Geometry: final body of the model. Coordinates: model frame, mm. A direction names the side the tool comes from. Coordinates: 2 decimals unless noted, no trailing zeros. Write each loop counter-clockwise with the first axis right and the second up, starting at its lowest first coordinate (ties: lowest second). Pieces come first, ordered by that corner, then holes. Notation, with made-up numbers: (-26.75, 8.25) - (13.25, 8.25) arc R18 cw to (13.25, 40.25) - close; hole circle Ø1 at (0, 51). An arc over 180 degrees is marked (long way). Answer as a JSON object with one key per item and string values. Group by question number.
Item 1: Line query: line 1 along Y through (x, z) = (8, 1.25); line 2 along X through (y, z) = (-14.5, 9.25); line 3 along Y through (x, z) = (1.5, 7.5). Output: solid intervals per line, ascending. Write a range as from..to.
Item 2: First-contact query: pin 1 Ø2 at (x, z) = (8.5, 7) entering from -Y; pin 2 Ø6.5 at (y, z) = (-8.5, 7) entering from +X. Flat tips, straight axial feed; report the tip coordinate or a pass-through.
Item 3: Mould query, pull axis Z, two halves, no side actions, for faces 3 (the flat face through (1, -5, 0)), 4 (the flat face through (0, -11.5, 4.8)), 5 (the cylindrical face through (0.867, -13.675, 4.249)). Classes: pulls with the +Z half, pulls with the -Z half, needs draft (parallel to the pull), parting line crosses it, or undercut.
Item 4: Set-up query: faces 1 (the flat face through (1.709, -10, 6)), 2 (the flat face through (10, 0, 6)). Return all of +Z, -Z, +X, -X, +Y, -Y with unobstructed straight access to the full face (end or side cutting, diameter ignored); none if empty.
Item 5: Section C-C on z = 12. Return loops of the section in (x, y).
Item 6: Section A-A on z = 6.35. Return loops of the section in (x, y), and give its area (3 significant figures).
Item 7: Section D-D on y = -16. Return loops of the section in (x, z).
Item 8: Section B-B on y = -11.75. Return loops of the section in (x, z).
```python
from build123d import *

# Parameters (mm, degrees)
F1_DEPTH = 12.7
F2_R     = 1.98374
F3_R     = 3.69316
F4_R     = 2.15265
F5_DEPTH = 1.70942
F6_R     = 2.15265
F7_DEPTH = 1.70942


with BuildPart() as f1:
    # F0 (on Top) → F1 (new body)
    with BuildSketch(Plane.XY):
        Polygon((19.558, 0), (0, 0), (0, -19.558), (1.70942, -19.558), (1.70942, -1.70942), (19.558, -1.70942), align=None)
    extrude(amount=F1_DEPTH)

    # F2
    f2_edges = [f1.edges().sort_by_distance(p)[0] for p in [
        (1.70942, -1.70942, 6.35),
    ]]
    fillet(f2_edges, radius=F2_R)

    # F3
    f3_edges = [f1.edges().sort_by_distance(p)[0] for p in [
        (0, 0, 6.35),
    ]]
    fillet(f3_edges, radius=F3_R)

    # F4 (on face) → F5 (cut, through all)
    with BuildSketch(Plane.XZ.offset(1.70942)):
        with Locations((13.208, 6.35)):
            Circle(F4_R)
    extrude(amount=-F5_DEPTH, mode=Mode.SUBTRACT)

    # F6 (on face) → F7 (cut, through all)
    with BuildSketch(Plane.YZ.offset(1.70942)):
        with Locations((-13.208, 6.35)):
            Circle(F6_R)
    extrude(amount=-F7_DEPTH, mode=Mode.SUBTRACT)


solid = f1.part
```
Checks:
{
 "1": {"line 1": "-1.71..0", "line 2": "0..1.71", "line 3": "-19.56..-15.03, -11.39..-0.72"},
 "2": {"pin 1": "y = -1.71", "pin 2": "x = 1.71"},
 "3": {"face 3": "pulls with the -Z half", "face 4": "needs draft", "face 5": "undercut"},
 "4": {"face 1": "+Z, -Z, +X, -Y", "face 2": "+Z, -Z, +X, -X, +Y"},
 "5": {"outline": "(0, -19.56) - (1.71, -19.56) - (1.71, -3.69) arc R1.98 cw to (3.69, -1.71) - (19.56, -1.71) - (19.56, 0) - (3.69, 0) arc R3.69 ccw to (0, -3.69) - close"},
 "6": {"outline": "(0, -19.56) - (1.71, -19.56) - (1.71, -15.36) - (0, -15.36) - close; (0, -11.06) - (1.71, -11.06) - (1.71, -3.69) arc R1.98 cw to (3.69, -1.71) - (11.06, -1.71) - (11.06, 0) - (3.69, 0) arc R3.69 ccw to (0, -3.69) - close; (15.36, -1.71) - (19.56, -1.71) - (19.56, 0) - (15.36, 0) - close", "area": "47.1 mm^2"},
 "7": {"outline": "(0, 0) - (1.71, 0) - (1.71, 12.7) - (0, 12.7) - close"},
 "8": {"outline": "(0, 0) - (1.71, 0) - (1.71, 4.77) - (0, 4.77) - close; (0, 7.93) - (1.71, 7.93) - (1.71, 12.7) - (0, 12.7) - close"}
}
